Geometry check sheet. Reference: the model listing, model coordinates, mm. A direction names the side the tool comes from. Coordinates: 2 decimals unless noted, no trailing zeros. Write each loop counter-clockwise with the first axis right and the second up, starting at its lowest first coordinate (ties: lowest second). Pieces come first, ordered by that corner, then holes.
from build123d import *

# Parameters (mm, degrees)
BOSS_EXTRUDE1_DEPTH          = 2
F_6_0_6_DIAMETER_HOLE1_D     = 6
F_6_0_6_DIAMETER_HOLE1_DEPTH = 25
F_5_0_5_DIAMETER_HOLE1_D     = 5
F_5_0_5_DIAMETER_HOLE1_DEPTH = 6.031754163


with BuildPart() as part:
    # Sketch1 → Revolve1 (revolve)
    with BuildSketch(Plane(origin=(0, 0, 0), x_dir=(-1, 0, 0), z_dir=(0, 0, -1)), mode=Mode.PRIVATE) as revolve1_sk:
        with BuildLine():
            Line((-29.5, 4), (-29.5, 0))
            Line((-29.5, 0), (29.5, 0))
            Line((29.5, 0), (29.5, 4))
            Line((29.5, 4), (28.25, 4))
            ThreePointArc((28.25, 4), (27.515753003, 4.754613948), (26.5, 5.031754163))
            Line((26.5, 5.031754163), (-26.5, 5.031754163))
            ThreePointArc((-26.5, 5.031754163), (-27.515753003, 4.754613948), (-28.25, 4))
            Line((-28.25, 4), (-29.5, 4))
        make_face()
    revolve(revolve1_sk.sketch.rotate(Axis((29.5, 0, 0), (-1, 0, 0)), 180), axis=Axis((29.5, 0, 0), (-1, 0, 0)))

    # Sketch2 → Boss-Extrude1 (add)
    with BuildSketch(Plane.XY.offset(1)):
        with BuildLine():
            Line((37.5, 3), (29.5, 3))
            Line((29.5, 3), (29.5, -3))
            Line((29.5, -3), (37.5, -3))
            ThreePointArc((37.5, -3), (40.5, 0), (37.5, 3))
        make_face()
    extrude(amount=-BOSS_EXTRUDE1_DEPTH)

    # 6.0 _6_ Diameter Hole1
    with Locations(Plane.ZY.offset(29.5)):
        with Locations((0, 0)):
            Hole(F_6_0_6_DIAMETER_HOLE1_D / 2, depth=F_6_0_6_DIAMETER_HOLE1_DEPTH)

    # 5.0 _5_ Diameter Hole1
    with Locations(Plane(origin=(0, 0, -1), x_dir=(-1, 0, 0), z_dir=(0, 0, -1))):
        with Locations((-37.5, 0)):
            Hole(F_5_0_5_DIAMETER_HOLE1_D / 2, depth=F_5_0_5_DIAMETER_HOLE1_DEPTH)


solid = part.part
1. Thickness scan on line 1 along Y through (x, z) = (37.5, 0.2); line 2 along Y through (x, z) = (-12.5, -2); line 3 along X through (y, z) = (-3.75, -0.75). Record the ranges inside material, lowest first.
Computed values:
line 1: y = -3 to -2.5, 2.5 to 3
line 2: y = -4.62 to -2.24, 2.24 to 4.62
line 3: x = -29.5 to 29.5
2. Sectioned sample at A-A, the plane y = 0. Record the boundary of the cut face in (x, z), and give its area (4 significant figures).
Computed values:
outline: (-29.5, -4) - (-28.25, -4) arc R2 ccw to (-26.5, -5.03) - (26.5, -5.03) arc R2 ccw to (28.25, -4) - (29.5, -4) - (29.5, -1) - (35, -1) - (35, 1) - (29.5, 1) - (29.5, 4) - (28.25, 4) arc R2 ccw to (26.5, 5.03) - (-26.5, 5.03) arc R2 ccw to (-28.25, 4) - (-29.5, 4) - (-29.5, 3) - (-4.5, 3) - (-4.5, -3) - (-29.5, -3) - close; (40, -1) - (40.5, -1) - (40.5, 1) - (40, 1) - close
area: 448.5 mm2
3. Gauge pin test, flat ends, axial feed: pin 1 Ø1 at (x, z) = (33, 0) entering from -Y; pin 2 Ø1 at (x, z) = (10, 1.5) entering from -Y; pin 3 Ø3 at (x, y) = (37.5, 0) entering from -Z; pin 4 Ø5 at (x, z) = (30.5, -3) entering from +Y. Record the tip position at first contact, or that the pin passes through.
Computed values:
pin 1: stops at y = -3
pin 2: stops at y = -4.93
pin 3: passes through
pin 4: stops at y = 3.94
4. Draft check along Z on faces 1 (the cylindrical face through (0.37, -4.8, 1.51)), 2 (the flat face through (34, 3, 0)), 3 (the cylindrical face through (-17, 0, 3)). Enter one of: released by +Z, released by -Z, zero draft, split by the parting line, or undercut.
Computed values:
face 1: split by the parting line
face 2: zero draft
face 3: undercut
5. Sectioned sample at C-C, the plane x = -23.5. Record the boundary of the cut face in (y, z).
Computed values:
outline: circle Ø10.06 at (0, 0); hole circle Ø6 at (0, 0)
6. Sectioned sample at B-B, the plane z = 0. Record the boundary of the cut face in (x, y).
Computed values:
outline: (-29.5, -4) - (-28.25, -4) arc R2 ccw to (-26.5, -5.03) - (26.5, -5.03) arc R2 ccw to (28.25, -4) - (29.5, -4) - (29.5, -3) - (37.5, -3) arc R3 ccw to (37.5, 3) - (29.5, 3) - (29.5, 4) - (28.25, 4) arc R2 ccw to (26.5, 5.03) - (-26.5, 5.03) arc R2 ccw to (-28.25, 4) - (-29.5, 4) - (-29.5, 3) - (-4.5, 3) - (-4.5, -3) - (-29.5, -3) - close; hole circle Ø5 at (37.5, 0)
7. Access from +Z, -Z, +X, -X, +Y, -Y to the whole of each face (thin tool, end or side, straight path). Record for faces 4 (the cylindrical face through (-28.866, 0.867, -3.905)), 5 (the flat face through (34, 0, -1)), 6 (the flat face through (33, -3, 0)).
Computed values:
face 4: -X
face 5: -Z, +X, +Y, -Y
face 6: +Z, -Z, +X, -Y
8. Sectioned sample at D-D, the plane x = -3.5. Record the boundary of the cut face in (y, z), and give its area (3 significant figures).
Computed values:
outline: circle Ø10.06 at (0, 0)
area: 79.5 mm2
